```python
from build123d import *

# Parameters (mm, degrees)
F0_W      = 177
F0_H      = 51
F1_DEPTH  = 7.5
F3_DEPTH  = 8
F4_DEPTH  = 0.8
F5_R      = 1.5
F6_DEPTH  = 3
F8_DEPTH  = 8
F9_DEPTH  = 0.8
F10_R     = 1.5
F11_DEPTH = 3
F12_SIZE  = 6


with BuildPart() as f1:
    # F0 (on Top) → F1 (new body)
    with BuildSketch(Plane.XY):
        Rectangle(F0_W, F0_H)
    extrude(amount=F1_DEPTH)

    # F2 (on face) → F3 (join)
    with BuildSketch(Plane.XZ.offset(25.5)):
        with BuildLine():
            ThreePointArc((77.25, 3.75), (76.1516504294, 6.4016504294), (73.5, 7.5))
            ThreePointArc((73.5, 7.5), (69.75, 3.75), (73.5, 0))
            ThreePointArc((73.5, 0), (76.1516504294, 1.0983495706), (77.25, 3.75))
        make_face()
        with BuildLine():
            ThreePointArc((-73.5, 0), (-70.8483495706, 1.0983495706), (-69.75, 3.75))
            ThreePointArc((-69.75, 3.75), (-70.8483495706, 6.4016504294), (-73.5, 7.5))
            ThreePointArc((-73.5, 7.5), (-77.25, 3.75), (-73.5, 0))
        make_face()
    extrude(amount=F3_DEPTH)

    # F2 (on face) → F4 (join)
    with BuildSketch(Plane.XZ.offset(25.5)):
        with BuildLine():
            ThreePointArc((-73.5, 0), (-77.25, 3.75), (-73.5, 7.5))
            Line((-73.5, 7.5), (-78.1837484988, 7.5))
            ThreePointArc((-78.1837484988, 7.5), (-79.5, 3.75), (-78.1837484988, 0))
            Line((-78.1837484988, 0), (-73.5, 0))
        make_face()
        with BuildLine():
            ThreePointArc((-73.5, 7.5), (-70.8483495706, 6.4016504294), (-69.75, 3.75))
            ThreePointArc((-69.75, 3.75), (-70.8483495706, 1.0983495706), (-73.5, 0))
            Line((-73.5, 0), (-68.8162515012, 0))
            ThreePointArc((-68.8162515012, 0), (-67.8386180577, 1.7628526719), (-67.5, 3.75))
            ThreePointArc((-67.5, 3.75), (-67.8386180577, 5.7371473281), (-68.8162515012, 7.5))
            Line((-68.8162515012, 7.5), (-73.5, 7.5))
        make_face()
        with BuildLine():
            ThreePointArc((79.5, 3.75), (79.1613819423, 5.7371473281), (78.1837484988, 7.5))
            Line((78.1837484988, 7.5), (73.5, 7.5))
            ThreePointArc((73.5, 7.5), (76.1516504294, 6.4016504294), (77.25, 3.75))
            ThreePointArc((77.25, 3.75), (76.1516504294, 1.0983495706), (73.5, 0))
            Line((73.5, 0), (78.1837484988, 0))
            ThreePointArc((78.1837484988, 0), (79.1613819423, 1.7628526719), (79.5, 3.75))
        make_face()
        with BuildLine():
            Line((73.5, 7.5), (68.8162515012, 7.5))
            ThreePointArc((68.8162515012, 7.5), (67.5, 3.75), (68.8162515012, 0))
            Line((68.8162515012, 0), (73.5, 0))
            ThreePointArc((73.5, 0), (69.75, 3.75), (73.5, 7.5))
        make_face()
    extrude(amount=F4_DEPTH)

    # F5 (on face) → F6 (cut)
    with BuildSketch(Plane.XZ.offset(33.5)):
        with Locations((-73.5, 3.75)):
            Circle(F5_R)
        with Locations((73.5, 3.75)):
            Circle(F5_R)
    extrude(amount=-F6_DEPTH, mode=Mode.SUBTRACT)

    # F7 (on face) → F8 (join)
    with BuildSketch(Plane(origin=(0, 25.5, 0), x_dir=(-1, 0, 0), z_dir=(0, 1, 0))):
        with BuildLine():
            ThreePointArc((77.25, 3.75), (76.1516504294, 6.4016504294), (73.5, 7.5))
            ThreePointArc((73.5, 7.5), (69.75, 3.75), (73.5, 0))
            ThreePointArc((73.5, 0), (76.1516504294, 1.0983495706), (77.25, 3.75))
        make_face()
        with BuildLine():
            ThreePointArc((-73.5, 0), (-70.8483495706, 1.0983495706), (-69.75, 3.75))
            ThreePointArc((-69.75, 3.75), (-70.8483495706, 6.4016504294), (-73.5, 7.5))
            ThreePointArc((-73.5, 7.5), (-77.25, 3.75), (-73.5, 0))
        make_face()
    extrude(amount=F8_DEPTH)

    # F7 (on face) → F9 (join)
    with BuildSketch(Plane(origin=(0, 25.5, 0), x_dir=(-1, 0, 0), z_dir=(0, 1, 0))):
        with BuildLine():
            Line((73.5, 7.5), (68.8162515012, 7.5))
            ThreePointArc((68.8162515012, 7.5), (67.5, 3.75), (68.8162515012, 0))
            Line((68.8162515012, 0), (73.5, 0))
            ThreePointArc((73.5, 0), (69.75, 3.75), (73.5, 7.5))
        make_face()
        with BuildLine():
            ThreePointArc((79.5, 3.75), (79.1613819423, 5.7371473281), (78.1837484988, 7.5))
            Line((78.1837484988, 7.5), (73.5, 7.5))
            ThreePointArc((73.5, 7.5), (76.1516504294, 6.4016504294), (77.25, 3.75))
            ThreePointArc((77.25, 3.75), (76.1516504294, 1.0983495706), (73.5, 0))
            Line((73.5, 0), (78.1837484988, 0))
            ThreePointArc((78.1837484988, 0), (79.1613819423, 1.7628526719), (79.5, 3.75))
        make_face()
        with BuildLine():
            ThreePointArc((-73.5, 0), (-77.25, 3.75), (-73.5, 7.5))
            Line((-73.5, 7.5), (-78.1837484988, 7.5))
            ThreePointArc((-78.1837484988, 7.5), (-79.5, 3.75), (-78.1837484988, 0))
            Line((-78.1837484988, 0), (-73.5, 0))
        make_face()
        with BuildLine():
            ThreePointArc((-73.5, 7.5), (-70.8483495706, 6.4016504294), (-69.75, 3.75))
            ThreePointArc((-69.75, 3.75), (-70.8483495706, 1.0983495706), (-73.5, 0))
            Line((-73.5, 0), (-68.8162515012, 0))
            ThreePointArc((-68.8162515012, 0), (-67.8386180577, 1.7628526719), (-67.5, 3.75))
            ThreePointArc((-67.5, 3.75), (-67.8386180577, 5.7371473281), (-68.8162515012, 7.5))
            Line((-68.8162515012, 7.5), (-73.5, 7.5))
        make_face()
    extrude(amount=F9_DEPTH)

    # F10 (on face) → F11 (cut)
    with BuildSketch(Plane(origin=(0, 33.5, 0), x_dir=(-1, 0, 0), z_dir=(0, 1, 0))):
        with Locations((-73.5, 3.75)):
            Circle(F10_R)
        with Locations((73.5, 3.75)):
            Circle(F10_R)
    extrude(amount=-F11_DEPTH, mode=Mode.SUBTRACT)

    # F12
    f12_edges = [f1.edges().sort_by_distance(p)[0] for p in [
        (-88.5, 0, 7.5),
    ]]
    chamfer(f12_edges, length=F12_SIZE)


solid = f1.part
```
Read the model definition and answer for the solid it produces. Units are mm, in the model's axes. A direction names the side the tool comes from. Coordinates: 2 decimals unless noted, no trailing zeros. Write each loop counter-clockwise with the first axis right and the second up, starting at its lowest first coordinate (ties: lowest second). Pieces come first, ordered by that corner, then holes. Notation, with made-up numbers: (32, 49) - (41, 49) arc R23 cw to (41, 83) - close; hole circle Ø3 at (-2.75, 88). An arc over 180 degrees is marked (long way). Answer as a JSON object with one key per item and string values. Group by question number.
1. A cutting plane is placed at B-B (x = -58). Determine the outline of the cut face in (y, z), plus the area to 4 significant figures.
2. Which of the six approach directions +Z, -Z, +X, -X, +Y, -Y give full straight-line access (tool end or side, diameter ignored) to faces 1 (the flat face through (-1, 25.5, 4)), 2 (the cylindrical face through (72.07, 32.02, 4.2)), 3 (the flat face through (-78, -26.3, 4)), 4 (the flat face through (78, 26.3, 4)), 5 (the flat face through (73, -30.5, 4))?
3. The mould has two halves that part along X. Classify faces 6 (the flat face through (83, 25.5, 4)), 7 (the flat face through (88.5, 0, 4)), 8 (the flat face through (-74, -30.5, 4)): +X half, -X half, draft (parallel to the pull), parting line (faces both ways), or undercut.
4. A cutting plane is placed at A-A (y = 28.5). Determine the outline of the cut face in (x, z).
5. Each of these flat-tipped pins is pushed along its axis until it touches: P1, Ø2, axis at x = 28, z = 4.5, coming from the +Y side; P2, Ø3.5, axis at x = 73, z = 4, coming from the +Y side; P3, Ø2.5, axis at x = 73.5, z = 3.75, coming from the +Y side. Where does it stop, or does it pass through?
6. Consider L1, parallel to Z at x = 73.5, y = 31.4; L2, parallel to X at y = -29, z = 3.5; L3, parallel to Y at x = -51, z = 4.5. Determine where each line is inside the solid, lowest interval first. Write a range as [from, to].
Worked out:
{
 "1": {"outline": "(-25.5, 0) - (25.5, 0) - (25.5, 7.5) - (-25.5, 7.5) - close", "area": "382.5 mm²"},
 "2": {"face 1": "+Z, -Z, +Y", "face 2": "+Y", "face 3": "-X, -Y", "face 4": "+X, +Y", "face 5": "-Y"},
 "3": {"face 6": "draft", "face 7": "+X half", "face 8": "undercut"},
 "4": {"outline": "circle Ø7.5 at (-73.5, 3.75); circle Ø7.5 at (73.5, 3.75)"},
 "5": {"P1": "stops at y = 25.5", "P2": "stops at y = 33.5", "P3": "stops at y = 30.5"},
 "6": {"L1": "z = [0, 2.25], [5.25, 7.5]", "L2": "x = [-77.24, -69.76], [69.76, 77.24]", "L3": "y = [-25.5, 25.5]"}
}
